from build123d import *

# Parameters (mm, degrees)
SKETCH1_W           = 4
SKETCH1_H           = 4
SKETCH1_R           = 2
SKETCH1_R_2         = 1
BOSS_EXTRUDE1_DEPTH = 2.5
FILLET1_R           = 2


with BuildPart() as part:
    # Sketch1 → Boss-Extrude1 (new body)
    # profile 1 of 9: a face of its own
    with BuildSketch(Plane(origin=(0, 0, 0), x_dir=(1, 0, 0), z_dir=(0, 1, 0))):
        Rectangle(SKETCH1_W, SKETCH1_H)
    # profile 2 of 9: a face of its own
    with BuildSketch(Plane(origin=(0, 0, 0), x_dir=(1, 0, 0), z_dir=(0, 1, 0))):
        with BuildLine():
            ThreePointArc((-4, 0), (-4.585786438, -1.414213562), (-6, -2))
            Line((-6, -2), (-2, -2))
            Line((-2, -2), (-2, 2))
            Line((-2, 2), (-6, 2))
            ThreePointArc((-6, 2), (-4.585786438, 1.414213562), (-4, 0))
        make_face()
    # profile 3 of 9: a face of its own
    with BuildSketch(Plane(origin=(0, 0, 0), x_dir=(1, 0, 0), z_dir=(0, 1, 0))):
        with Locations((-6, 0)):
            Circle(SKETCH1_R)
        with Locations(Location((-6, 0, 0), (0, 0, 270))):
            Circle(SKETCH1_R_2, mode=Mode.SUBTRACT)
    # profile 4 of 9: a face of its own
    with BuildSketch(Plane(origin=(0, 0, 0), x_dir=(1, 0, 0), z_dir=(0, 1, 0))):
        with Locations((0, -6)):
            Circle(SKETCH1_R)
        with Locations(Location((0, -6, 0), (0, 0, 270))):
            Circle(SKETCH1_R_2, mode=Mode.SUBTRACT)
    # profile 5 of 9: a face of its own
    with BuildSketch(Plane(origin=(0, 0, 0), x_dir=(1, 0, 0), z_dir=(0, 1, 0))):
        with BuildLine():
            Line((2, -2), (-2, -2))
            Line((-2, -2), (-2, -6))
            ThreePointArc((-2, -6), (0, -4), (2, -6))
            Line((2, -6), (2, -2))
        make_face()
    # profile 6 of 9: a face of its own
    with BuildSketch(Plane(origin=(0, 0, 0), x_dir=(1, 0, 0), z_dir=(0, 1, 0))):
        with BuildLine():
            Line((-2, 6), (-2, 2))
            Line((-2, 2), (2, 2))
            Line((2, 2), (2, 6))
            ThreePointArc((2, 6), (0, 4), (-2, 6))
        make_face()
    # profile 7 of 9: a face of its own
    with BuildSketch(Plane(origin=(0, 0, 0), x_dir=(1, 0, 0), z_dir=(0, 1, 0))):
        with Locations((0, 6)):
            Circle(SKETCH1_R)
        with Locations(Location((0, 6, 0), (0, 0, 270))):
            Circle(SKETCH1_R_2, mode=Mode.SUBTRACT)
    # profile 8 of 9: a face of its own
    with BuildSketch(Plane(origin=(0, 0, 0), x_dir=(1, 0, 0), z_dir=(0, 1, 0))):
        with BuildLine():
            Line((2, 2), (2, -2))
            Line((2, -2), (6, -2))
            ThreePointArc((6, -2), (4, 0), (6, 2))
            Line((6, 2), (2, 2))
        make_face()
    # profile 9 of 9: a face of its own
    with BuildSketch(Plane(origin=(0, 0, 0), x_dir=(1, 0, 0), z_dir=(0, 1, 0))):
        with Locations((6, 0)):
            Circle(SKETCH1_R)
        with Locations(Location((6, 0, 0), (0, 0, 270))):
            Circle(SKETCH1_R_2, mode=Mode.SUBTRACT)
    extrude(amount=BOSS_EXTRUDE1_DEPTH)

    # Fillet1
    fillet1_edges = [part.edges().sort_by_distance(p)[0] for p in [
        (-2, 1.25, -2),
        (2, 1.25, -2),
        (2, 1.25, 2),
        (-2, 1.25, 2),
    ]]
    fillet(fillet1_edges, radius=FILLET1_R)

    # Sketch3 → Revolve1 (revolve)
    with BuildSketch(Plane.XY, mode=Mode.PRIVATE) as revolve1_sk:
        Polygon((0, 2.5), (3.5, 2.5), (3.5, 5), (9.65, 5), (9.65, 16), (3, 18.5), (3, 32.5), (0, 32.5), align=None)
    revolve(revolve1_sk.sketch.rotate(Axis((0, 2.5, 0), (0, 1, 0)), 90), axis=Axis((0, 2.5, 0), (0, 1, 0)))


solid = part.part
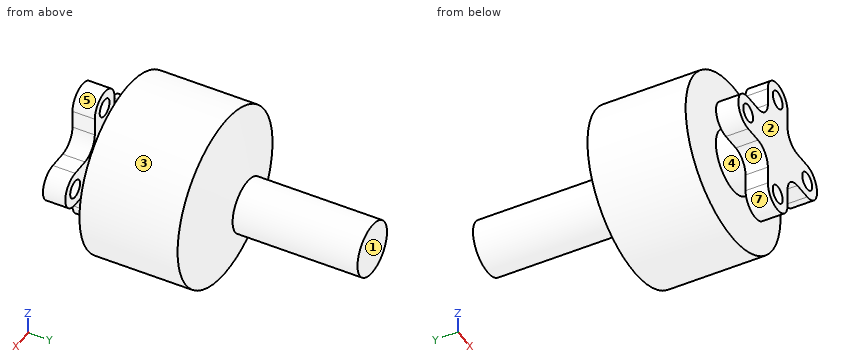
Part model, mm, in its own coordinate system. Face numbers are marked on the shaded views. A direction names the side the tool comes from. Round coordinates to 2 decimals unless told otherwise and drop trailing zeros. Order: outer loops, then holes, each group sorted by start corner. A loop starts at its lowest first (then second) coordinate and runs counter-clockwise, first axis right, second up. Notation, with made-up numbers: (-24, 12) -> (33, 12) arc R18 cw to (33, 42) -> close; hole circle Ø6 at (53, 73). An arc over 180 degrees is marked (long way). Put each result on its own line as item: value.
Q1. Tool access for the marked faces 5, 6 and 7: list every direction of +Z, -Z, +X, -X, +Y, -Y with a clear straight run to the whole face (end or side of a thin tool).
From the geometry:
face 5: +Z, -Y
face 6: -Z, -X, -Y
face 7: -Z, -Y
Q2. Pin check, flat tips, straight feed: pin 1 Ø1 at (x, y) = (4.5, 0.5) entering from -Z; pin 2 Ø4 at (x, y) = (6, 11.5) entering from -Z; pin 3 Ø1 at (y, z) = (1, -5.5) entering from -X. Stop position of each tip, or through.
From the geometry:
pin 1: stops at z = -2
pin 2: stops at z = -8.78
pin 3: stops at x = -2
Q3. Band-saw the part on D-D (y = 15). Give the cut face in (x, z).
From the geometry:
outline: circle Ø19.3 at (0, 0)
Q4. Band-saw the part on C-C (x = 0). Give the cut face in (y, z).
From the geometry:
outline: (0, -8) -> (2.5, -8) -> (2.5, -7) -> (0, -7) -> close; (0, -5) -> (2.5, -5) -> (2.5, -3.5) -> (5, -3.5) -> (5, -9.65) -> (16, -9.65) -> (18.5, -3) -> (32.5, -3) -> (32.5, 3) -> (18.5, 3) -> (16, 9.65) -> (5, 9.65) -> (5, 3.5) -> (2.5, 3.5) -> (2.5, 5) -> (0, 5) -> close; (0, 7) -> (2.5, 7) -> (2.5, 8) -> (0, 8) -> close
Q5. Band-saw the part on B-B (y = 2). Give the cut face in (x, z).
From the geometry:
outline: (-6, -2) -> (-4, -2) arc R2 cw to (-2, -4) -> (-2, -6) arc R2 ccw to (2, -6) -> (2, -4) arc R2 cw to (4, -2) -> (6, -2) arc R2 ccw to (6, 2) -> (4, 2) arc R2 cw to (2, 4) -> (2, 6) arc R2 ccw to (-2, 6) -> (-2, 4) arc R2 cw to (-4, 2) -> (-6, 2) arc R2 ccw to start; hole circle Ø2 at (-6, 0); hole circle Ø2 at (0, -6); hole circle Ø2 at (0, 6); hole circle Ø2 at (6, 0)
Q6. Wall check: line 1 (X direction, y = 1.45, z = 0); line 2 (X direction, y = 7, z = -0.25); line 3 (Y direction, x = 0.5, z = -4.75). Give the ranges that are in metal, low to high. Write a range as [from, to].
From the geometry:
line 1: x = [-8, -7], [-5, 5], [7, 8]
line 2: x = [-9.65, 9.65]
line 3: y = [0, 2.5], [5, 17.83]
Q7. Pull direction Y, two halves, no side cores. Call the marked faces 1, 2, 3 and 4: pulls with the +Y half, pulls with the -Y half, needs draft (parallel to the pull), parting line crosses it, or undercut.
From the geometry:
face 1: pulls with the +Y half
face 2: pulls with the -Y half
face 3: needs draft
face 4: undercut
Q8. Band-saw the part on A-A (z = 0). Give the cut face in (x, y), and give its area (3 significant figures).
From the geometry:
outline: (-9.65, 5) -> (-3.5, 5) -> (-3.5, 2.5) -> (-5, 2.5) -> (-5, 0) -> (5, 0) -> (5, 2.5) -> (3.5, 2.5) -> (3.5, 5) -> (9.65, 5) -> (9.65, 16) -> (3, 18.5) -> (3, 32.5) -> (-3, 32.5) -> (-3, 18.5) -> (-9.65, 16) -> close; (-8, 0) -> (-7, 0) -> (-7, 2.5) -> (-8, 2.5) -> close; (7, 0) -> (8, 0) -> (8, 2.5) -> (7, 2.5) -> close
area: 375 mm2
